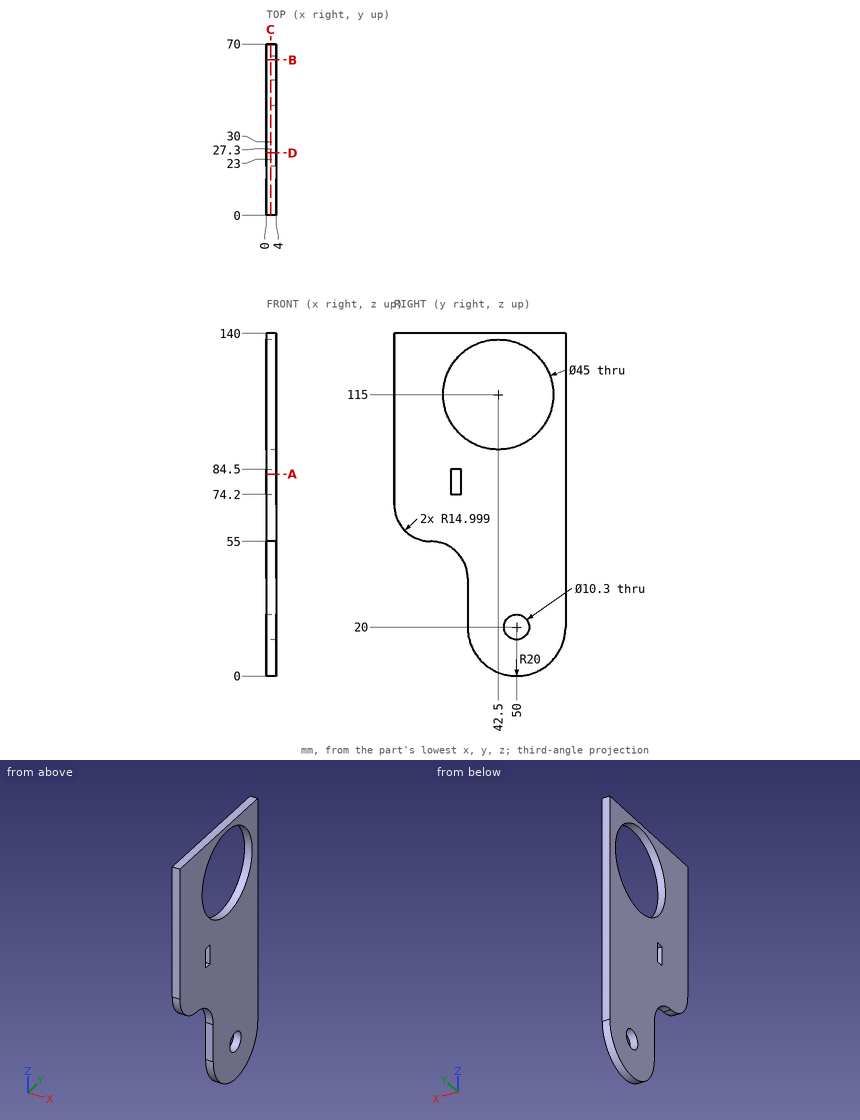
Design review of the part shown in the three views and the two pictorial views. Dimensions are in mm from the part's minimum x, y and z. Give positions to 0.01 mm unless a question says otherwise; leave off trailing zeros. Write each loop counter-clockwise with the first axis right and the second up, starting at its lowest first coordinate (ties: lowest second). Pieces come first, ordered by that corner, then holes.
Item 1: Take a section at D-D (y = 25.5). Give the boundary of the cut face in (x, z), and give its area (3 significant figures).
Item 2: Take a section at C-C (x = 1.75). Give the number of separate pieces and of enclosed holes in the cut face, and give its area (3 significant figures).
Item 3: Wall thickness on probe 1 along Z at (x, y) = (0.6, 46) (1 decimal); probe 2 along Y at (x, z) = (2.15, 20); probe 3 along Z at (x, y) = (2.6, 25.5) (1 decimal): over which ranges is each line inside the solid? List them lowest first.
Item 4: Insertion check: P1, Ø2, axis at x = 1.5, z = 38, coming from the -Y side; P2, Ø2, axis at x = 2.5, z = 18, coming from the +Y side (1 decimal). Each pin has a flat end and moves straight along its axis. Give the tip position at first contact, or say it passes through.
Item 5: Take a section at B-B (y = 63.5). Give the boundary of the cut face in (x, z).
Item 6: Take a section at A-A (z = 82.5). Give the boundary of the cut face in (x, y), and give its area (3 significant figures).
Established:
1. outline: (0, 50.71) - (4, 50.71) - (4, 74.2) - (0, 74.2) - close; (0, 84.5) - (4, 84.5) - (4, 100.26) - (0, 100.26) - close; (0, 129.74) - (4, 129.74) - (4, 140) - (0, 140) - close
1. area: 198 mm2
2. separate pieces: 1
2. enclosed holes: 3
2. area: 6,260 mm2
3. probe 1: z = 0.4 to 16.8, 23.2 to 92.8, 137.2 to 140
3. probe 2: y = 30 to 44.85, 55.15 to 70
3. probe 3: z = 50.7 to 74.2, 84.5 to 100.3, 129.7 to 140
4. P1: stops at y = 30
4. P2: stops at y = 70
5. outline: (0, 5.24) - (4, 5.24) - (4, 106.92) - (0, 106.92) - close; (0, 123.08) - (4, 123.08) - (4, 140) - (0, 140) - close
6. outline: (0, 0) - (4, 0) - (4, 23) - (0, 23) - close; (0, 27.3) - (4, 27.3) - (4, 70) - (0, 70) - close
6. area: 263 mm2
